from build123d import *
from build123d.topology import SkipClean

# Parameters (mm, degrees)
SKETCH1_R           = 25
SKETCH1_R_2         = 17.5
BOSS_EXTRUDE1_DEPTH = 10
BOSS_EXTRUDE2_START = 10
SKETCH2_R           = 45
SKETCH2_R_2         = 5.6
SKETCH2_R_3         = 17.5
BOSS_EXTRUDE2_DEPTH = 10
CHAMFER1_SIZE       = 5
BOSS_EXTRUDE4_START = -20
SKETCH4_R           = 17.5
SKETCH4_R_2         = 16
BOSS_EXTRUDE4_DEPTH = 20
BOSS_EXTRUDE5_START = -20
SKETCH5_R           = 16
SKETCH5_R_2         = 15
BOSS_EXTRUDE5_DEPTH = 13
CHAMFER3_SIZE       = 10
SKETCH7_R           = 25
SKETCH7_R_2         = 16
BOSS_EXTRUDE6_DEPTH = 1
SKETCH8_R           = 16
SKETCH8_R_2         = 15
BOSS_EXTRUDE7_DEPTH = 1
SKETCH9_R           = 26
BOSS_EXTRUDE8_DEPTH = 1
CUT_EXTRUDE1_START  = -18
SKETCH10_R          = 15
CUT_EXTRUDE1_DEPTH  = 18
CHAMFER4_SIZE       = 3
SKETCH11_R          = 3.5
CUT_EXTRUDE2_DEPTH  = 5


with BuildPart() as part:
    # Sketch1 → Boss-Extrude1 (new body)
    with BuildSketch(Plane(origin=(0, 0, 0), x_dir=(1, 0, 0), z_dir=(0, 1, 0))):
        with Locations(Location((0, 0, 0), (0, 0, 270))):
            Circle(SKETCH1_R)
        with Locations(Location((0, 0, 0), (0, 0, 270))):
            Circle(SKETCH1_R_2, mode=Mode.SUBTRACT)
    extrude(amount=BOSS_EXTRUDE1_DEPTH)

    # Sketch2 → Boss-Extrude2 (add)
    with SkipClean():  # the faces are left unmerged after this step: merging them gives an invalid solid
        with BuildSketch(Plane.XZ.offset(BOSS_EXTRUDE2_START)):
            with Locations(Location((0, 0, 0), (0, 0, 270))):
                Circle(SKETCH2_R)
            with Locations(Location((35, 0, 0), (0, 0, 270))):
                Circle(SKETCH2_R_2, mode=Mode.SUBTRACT)
            with Locations(Location((24.748737342, -24.748737342, 0), (0, 0, 270))):
                Circle(SKETCH2_R_2, mode=Mode.SUBTRACT)
            with Locations(Location((0, -35, 0), (0, 0, 270))):
                Circle(SKETCH2_R_2, mode=Mode.SUBTRACT)
            with Locations(Location((-24.748737342, -24.748737342, 0), (0, 0, 270))):
                Circle(SKETCH2_R_2, mode=Mode.SUBTRACT)
            with Locations(Location((-35, 0, 0), (0, 0, 270))):
                Circle(SKETCH2_R_2, mode=Mode.SUBTRACT)
            with Locations(Location((-24.748737342, 24.748737342, 0), (0, 0, 270))):
                Circle(SKETCH2_R_2, mode=Mode.SUBTRACT)
            with Locations(Location((0, 35, 0), (0, 0, 270))):
                Circle(SKETCH2_R_2, mode=Mode.SUBTRACT)
            with Locations(Location((24.748737342, 24.748737342, 0), (0, 0, 270))):
                Circle(SKETCH2_R_2, mode=Mode.SUBTRACT)
            with Locations(Location((0, 0, 0), (0, 0, 270))):
                Circle(SKETCH2_R_3, mode=Mode.SUBTRACT)
        extrude(amount=-BOSS_EXTRUDE2_DEPTH)

    # Chamfer1
    # the kernel refuses this chamfer: 5 mm, written as the material it takes off along each edge
    with BuildSketch(Plane(origin=(0, 0, 0), x_dir=(0, 0, -1), z_dir=(-1, 0, 0))) as chamfer1_piece_1:
        Polygon((45 - CHAMFER1_SIZE, 0), (45, CHAMFER1_SIZE), (45, 0), align=None)
    revolve(axis=Axis((0, 0, 0), (0, -1, 0)), mode=Mode.SUBTRACT)

    # Sketch4 → Boss-Extrude4 (add)
    with BuildSketch(Plane(origin=(0, 10, 0), x_dir=(1, 0, 0), z_dir=(0, 1, 0)).offset(BOSS_EXTRUDE4_START)):
        Circle(SKETCH4_R)
        with Locations(Location((0, 0, 0), (0, 0, 270))):
            Circle(SKETCH4_R_2, mode=Mode.SUBTRACT)
    extrude(amount=BOSS_EXTRUDE4_DEPTH)

    # Sketch5 → Boss-Extrude5 (add)
    with BuildSketch(Plane(origin=(0, 10, 0), x_dir=(1, 0, 0), z_dir=(0, 1, 0)).offset(BOSS_EXTRUDE5_START)):
        with Locations(Location((0, 0, 0), (0, 0, 270))):
            Circle(SKETCH5_R)
        with Locations(Location((0, 0, 0), (0, 0, 270))):
            Circle(SKETCH5_R_2, mode=Mode.SUBTRACT)
    extrude(amount=BOSS_EXTRUDE5_DEPTH)

    # Chamfer3
    chamfer3_edges = [part.edges().sort_by_distance(p)[0] for p in [
        (0, -10, -15),
    ]]
    chamfer(chamfer3_edges, length=CHAMFER3_SIZE)

    # Sketch7 → Boss-Extrude6 (add)
    with BuildSketch(Plane(origin=(0, 10, 0), x_dir=(1, 0, 0), z_dir=(0, 1, 0))):
        with Locations(Location((0, 0, 0), (0, 0, 270))):
            Circle(SKETCH7_R)
        with Locations(Location((0, 0, 0), (0, 0, 270))):
            Circle(SKETCH7_R_2, mode=Mode.SUBTRACT)
    extrude(amount=BOSS_EXTRUDE6_DEPTH)

    # Sketch8 → Boss-Extrude7 (add)
    with BuildSketch(Plane(origin=(0, 3, 0), x_dir=(1, 0, 0), z_dir=(0, 1, 0))):
        with Locations(Location((0, 0, 0), (0, 0, 270))):
            Circle(SKETCH8_R)
        with Locations(Location((0, 0, 0), (0, 0, 270))):
            Circle(SKETCH8_R_2, mode=Mode.SUBTRACT)
    extrude(amount=BOSS_EXTRUDE7_DEPTH)

    # Sketch9 → Boss-Extrude8 (add)
    with BuildSketch(Plane(origin=(0, 0, 0), x_dir=(1, 0, 0), z_dir=(0, 1, 0))):
        with Locations(Location((0, 0, 0), (0, 0, 90))):
            Circle(SKETCH9_R)
    extrude(amount=BOSS_EXTRUDE8_DEPTH)

    # Sketch10 → Cut-Extrude1 (cut)
    with BuildSketch(Plane(origin=(0, 1, 0), x_dir=(1, 0, 0), z_dir=(0, 1, 0)).offset(CUT_EXTRUDE1_START)):
        with Locations(Location((0, 0, 0), (0, 0, 270))):
            Circle(SKETCH10_R)
    extrude(amount=CUT_EXTRUDE1_DEPTH, mode=Mode.SUBTRACT)

    # Chamfer4
    chamfer4_edges = [part.edges().sort_by_distance(p)[0] for p in [
        (-35, -10, 5.6),
        (-24.748737342, -10, 30.348737342),
        (0, -10, 40.6),
        (24.748737342, -10, 30.348737342),
        (35, -10, 5.6),
        (24.748737342, -10, -19.148737342),
        (0, -10, -29.4),
        (-24.748737342, -10, -19.148737342),
    ]]
    chamfer(chamfer4_edges, length=CHAMFER4_SIZE)

    # Sketch11 → Cut-Extrude2 (cut)
    with BuildSketch(Plane(origin=(0, 11, 0), x_dir=(1, 0, 0), z_dir=(0, 1, 0))):
        with Locations(Location((-20.5, 0, 0), (0, 0, 270))):
            Circle(SKETCH11_R)
        with Locations(Location((-14.495689014, 14.495689014, 0), (0, 0, 270))):
            Circle(SKETCH11_R)
        with Locations(Location((0, 20.5, 0), (0, 0, 270))):
            Circle(SKETCH11_R)
        with Locations(Location((14.495689014, 14.495689014, 0), (0, 0, 270))):
            Circle(SKETCH11_R)
        with Locations(Location((20.5, 0, 0), (0, 0, 270))):
            Circle(SKETCH11_R)
        with Locations(Location((14.495689014, -14.495689014, 0), (0, 0, 270))):
            Circle(SKETCH11_R)
        with Locations(Location((0, -20.5, 0), (0, 0, 270))):
            Circle(SKETCH11_R)
        with Locations(Location((-14.495689014, -14.495689014, 0), (0, 0, 270))):
            Circle(SKETCH11_R)
    extrude(amount=-CUT_EXTRUDE2_DEPTH, mode=Mode.SUBTRACT)


solid = part.part
Geometry check sheet. Reference: the model listing, model coordinates, mm. A direction names the side the tool comes from. Give positions to 0.01 mm unless a question says otherwise; leave off trailing zeros. Loops run counter-clockwise (first coordinate to the right, second up) from the corner with the lowest first, then second, coordinate; pieces in that order, holes last. Notation, with made-up numbers: M 73,37.5 L 104,37.5 A17 cw 104,47.5 Z; hole C 42.5,9.25 d8. An arc over 180 degrees is marked long. Write each question's results on one line, items separated by ' | '.
1) Thickness scan on line 1 (X direction, y = 3.25, z = 0); line 2 (Z direction, x = -3, y = 8.25); line 3 (Z direction, x = -21, y = -1.5). Record the ranges inside material, lowest first.
Answers follow:
line 1: -25 to -15, 15 to 25 | line 2: -24.82 to -22.3, -18.7 to -15.72, 15.72 to 18.7, 22.3 to 24.82 | line 3: -35.79 to -28.91, -20.59 to 20.59, 28.91 to 35.79
2) Release check for a two-part mould opening along Z. For faces 3 (the face through (15.821, 0.493, 20.633)), 4 (the face through (22.548, -7.146, 19.441)), 5 (the face through (-21, 1, 14)) record: +Z half, -Z half, draft (parallel to the pull), parting line (faces both ways), or undercut.
Answers follow:
face 3: parting line | face 4: undercut | face 5: draft
3) Gauge pin test, flat ends, axial feed: pin 1 (2 mm diameter, centred on y = 0.5, z = -21, fed in from +X); pin 2 (2 mm diameter, centred on x = 19.5, z = -1.5, fed in from +Y); pin 3 (14.5 mm diameter, centred on x = -35, z = 0, fed in from +Y). Record the tip position at first contact, or that the pin passes through.
Answers follow:
pin 1: x = 34.77 | pin 2: y = 6 | pin 3: y = 0
4) Section check A-A, the plane x = 0. Count the separate pieces of the cut face and the enclosed holes in it, plus the area to 3 significant figures.
Answers follow:
separate pieces: 4 | enclosed holes: 0 | area: 371 mm2
5) Tool access check on faces 1 (the face through (0.246, -3.549, -29.405)), 2 (the face through (15, 6, 14)). Record the directions out of +Z, -Z, +X, -X, +Y, -Y that give a thin tool (end or side, any length) a straight path to the whole face; none if there is none.
Answers follow:
face 1: +Y, -Y | face 2: +Y
6) Section check D-D, the plane y = 2.5. Record the boundary of the cut face in (x, z), plus the area to 3 significant figures.
Answers follow:
outline: C 0,0 d50; hole C 0,0 d30 | area: 1,260 mm2
